```python
from build123d import *

# Parameters (mm, degrees)
SKETCH1_R               = 19.05
BOSS_EXTRUDE1_DEPTH     = 10.16
SKETCH2_R               = 6.35
CUT_EXTRUDE1_DEPTH      = 15.494
SKETCH6_W               = 12.7
SKETCH6_H               = 12.7
BOSS_EXTRUDE6_DEPTH     = 10.16
BOSS_EXTRUDE7_START     = -10.16
BOSS_EXTRUDE7_DEPTH     = 10.16
CIRPATTERN7_START       = -6.35
CIRPATTERN7_OUTLINE_W   = 10.16
CIRPATTERN7_OUTLINE_H   = 12.7
CIRPATTERN7_DEPTH       = 12.7
CIRPATTERN7_START_2     = -19.05
CIRPATTERN7_2_OUTLINE_W = 10.16
CIRPATTERN7_2_OUTLINE_H = 12.7
CIRPATTERN7_2_DEPTH     = 1.089487758
CIRPATTERN7_START_3     = 17.960512242
CIRPATTERN7_3_OUTLINE_W = 10.16
CIRPATTERN7_3_OUTLINE_H = 12.7
CIRPATTERN7_3_DEPTH     = 1.089487758
SKETCH7_W               = 12.7
SKETCH7_H               = 10.16
BOSS_EXTRUDE9_DEPTH     = 12.7
SKETCH10_W              = 12.7
SKETCH10_H              = 10.16
BOSS_EXTRUDE10_DEPTH    = 12.7
SKETCH11_W              = 12.7
SKETCH11_H              = 10.16
BOSS_EXTRUDE11_DEPTH    = 12.7
SKETCH12_R              = 3.302
CUT_EXTRUDE3_DEPTH      = 16.256
CIRPATTERN8_COUNT       = 4


# Read off the part's stored shape, not the designer's step: CirPattern7
with BuildPart() as part:
    # Sketch1 → Boss-Extrude1 (new body)
    with BuildSketch(Plane(origin=(0, 0, 0), x_dir=(1, 0, 0), z_dir=(0, 1, 0))):
        with Locations(Location((0, 0, 0), (0, 0, 270))):
            Circle(SKETCH1_R)
    extrude(amount=BOSS_EXTRUDE1_DEPTH)

    # Sketch2 → Cut-Extrude1 (cut)
    with BuildSketch(Plane(origin=(0, 10.16, 0), x_dir=(1, 0, 0), z_dir=(0, 1, 0))):
        with Locations(Location((0, 0, 0), (0, 0, 270))):
            Circle(SKETCH2_R)
    extrude(amount=-CUT_EXTRUDE1_DEPTH, mode=Mode.SUBTRACT)



with BuildPart() as body_2:
    # Sketch6 → Boss-Extrude6 (new body)
    with BuildSketch(Plane(origin=(0, 10.16, 0), x_dir=(1, 0, 0), z_dir=(0, 1, 0))):
        with Locations((0, -25.4)):
            Rectangle(SKETCH6_W, SKETCH6_H)
    extrude(amount=-BOSS_EXTRUDE6_DEPTH)


with BuildPart() as part_1:
    add(part.part)

    add(body_2.part)  # Boss-Extrude7 merges body 2
    # Sketch6<4> → Boss-Extrude7 (add)
    with BuildSketch(Plane(origin=(0, 10.16, 0), x_dir=(1, 0, 0), z_dir=(0, 1, 0)).offset(BOSS_EXTRUDE7_START)):
        with BuildLine():
            Line((-6.35, -17.960512242), (-6.35, -19.05))
            Line((-6.35, -19.05), (0, -19.05))
            ThreePointArc((0, -19.05), (-3.221392695, -18.775652561), (-6.35, -17.960512242))
        make_face()
        with BuildLine():
            ThreePointArc((6.35, -17.960512242), (3.221392695, -18.775652561), (0, -19.05))
            Line((0, -19.05), (6.35, -19.05))
            Line((6.35, -19.05), (6.35, -17.960512242))
        make_face()
    extrude(amount=BOSS_EXTRUDE7_DEPTH)

    # CirPattern7 outline → CirPattern7 (add)
    with BuildSketch(Plane.YZ.offset(CIRPATTERN7_START)):
        with Locations((5.08, -12.7)):
            Rectangle(CIRPATTERN7_OUTLINE_W, CIRPATTERN7_OUTLINE_H)
    extrude(amount=CIRPATTERN7_DEPTH)

    # CirPattern7 2 outline → CirPattern7 2 (add)
    with BuildSketch(Plane.YZ.offset(CIRPATTERN7_START_2)):
        with Locations((5.08, 0)):
            Rectangle(CIRPATTERN7_2_OUTLINE_W, CIRPATTERN7_2_OUTLINE_H)
    extrude(amount=CIRPATTERN7_2_DEPTH)

    # CirPattern7 3 outline → CirPattern7 3 (add)
    with BuildSketch(Plane.YZ.offset(CIRPATTERN7_START_3)):
        with Locations((5.08, 0)):
            Rectangle(CIRPATTERN7_3_OUTLINE_W, CIRPATTERN7_3_OUTLINE_H)
    extrude(amount=CIRPATTERN7_3_DEPTH)

    # Sketch7 → Boss-Extrude9 (add)
    with BuildSketch(Plane.ZY.offset(19.05)):
        with Locations((0, 5.08)):
            Rectangle(SKETCH7_W, SKETCH7_H)
    extrude(amount=BOSS_EXTRUDE9_DEPTH)

    # Sketch10 → Boss-Extrude10 (add)
    with BuildSketch(Plane(origin=(19.05, 0, 0), x_dir=(0, 0, -1), z_dir=(1, 0, 0))):
        with Locations((0, 5.08)):
            Rectangle(SKETCH10_W, SKETCH10_H)
    extrude(amount=BOSS_EXTRUDE10_DEPTH)

    # Sketch11 → Boss-Extrude11 (add)
    with BuildSketch(Plane(origin=(0, 0, -19.05), x_dir=(-1, 0, 0), z_dir=(0, 0, -1))):
        with Locations((0, 5.08)):
            Rectangle(SKETCH11_W, SKETCH11_H)
    extrude(amount=BOSS_EXTRUDE11_DEPTH)

    # Sketch12 → Cut-Extrude3 (cut)
    with BuildSketch(Plane.XY.offset(6.35)):
        with Locations((26.67, 5.08)):
            Circle(SKETCH12_R)
    cut_extrude3 = extrude(amount=-CUT_EXTRUDE3_DEPTH, mode=Mode.SUBTRACT)

    # CirPattern8: Cut-Extrude3 ×4 about axis
    cirpattern8_axis = Axis((0, 0, 0), (0, -1, 0))
    for i in range(1, CIRPATTERN8_COUNT):
        add(cut_extrude3.rotate(cirpattern8_axis, i * 360 / CIRPATTERN8_COUNT), mode=Mode.SUBTRACT)


solid = part_1.part
```
Check sheet for the modelled part. Datum: model origin and axes. Units: mm. A direction names the side the tool comes from. Round coordinates to 2 decimals unless told otherwise and drop trailing zeros. Loops run counter-clockwise (first coordinate to the right, second up) from the corner with the lowest first, then second, coordinate; pieces in that order, holes last. Notation, with made-up numbers: (-31.5, 19) - (-20.5, 19) arc R17 ccw to (-20.5, 42) - close; hole circle Ø10 at (-37, 56.5). An arc over 180 degrees is marked (long way). Answer as a JSON object with one key per item and string values. Group by question number.
Q1. Sectioned sample at C-C, the plane z = 0. Enter the section's corners in (x, y).
Q2. Mould release check, pull along X, two halves, no side actions. Record for faces 6 (the face through (6.35, 6, 23)), 7 (the face through (23.37, 5.23, 0.09)), 8 (the face through (-0.09, 5.23, 23.37)): released by +X, released by -X, zero draft, split by the parting line, or undercut.
Q3. Set-up check for faces 1 (the face through (-23, 5, 6.35)), 2 (the face through (23, 5, 6.35)), 3 (the face through (-5, 10.16, 5)), 4 (the face through (-6.35, 5, -23)), 5 (the face through (13.55, 5.01, -13.39)): record each of +Z, -Z, +X, -X, +Y, -Y from which the full face is reachable in a straight line by a thin tool's end or side.
Q4. Sectioned sample at A-A, the plane y = 5.08. Count the separate pieces of the cut face and the enclosed holes in it, plus the area to 3 significant figures.
Q5. Scan lines: line 1 along Z through (x, y) = (0, 2.5); line 2 along Y through (x, z) = (0.75, -26.67); line 3 along X through (y, z) = (3, 0). Record each from-to range of solid material in increasing order. Write a range as [from, to].
Q6. Sectioned sample at D-D, the plane z = 26.67. Enter the section's corners in (x, y), plus the area to 3 significant figures.
Q7. Sectioned sample at B-B, the plane x = 0. Enter the section's corners in (y, z), plus the area to 3 significant figures.
Q8. Gauge pin test, flat ends, axial feed: P1, Ø5, axis at x = 25.5, y = 3.5, coming from the +Z side; P2, Ø2, axis at x = 24, y = 9, coming from the -Z side; P3, Ø5, axis at y = 6.5, z = 25.5, coming from the +X side. Record the tip position at first contact, or that the pin passes through.
Solution:
{
 "1": {"outline": "(-31.75, 0) - (-6.35, 0) - (-6.35, 10.16) - (-31.75, 10.16) - close; (6.35, 0) - (31.75, 0) - (31.75, 10.16) - (6.35, 10.16) - close; hole circle Ø6.6 at (-26.67, 5.08); hole circle Ø6.6 at (26.67, 5.08)"},
 "2": {"face 6": "released by +X", "face 7": "undercut", "face 8": "zero draft"},
 "3": {"face 1": "+Z, -X, +Y, -Y", "face 2": "+Z, +X, +Y, -Y", "face 3": "+Z, -Z, +X, -X, +Y", "face 4": "-Z, -X, +Y, -Y", "face 5": "-Z, +X, +Y, -Y"},
 "4": {"separate pieces": "5", "enclosed holes": "1", "area": "1,340 mm²"},
 "5": {"line 1": "z = [-31.75, -28.73], [-24.61, -6.35], [6.35, 24.61], [28.73, 31.75]", "line 2": "y = [0, 1.78], [8.38, 10.16]", "line 3": "x = [-31.75, -29.23], [-24.11, -6.35], [6.35, 24.11], [29.23, 31.75]"},
 "6": {"outline": "(-6.35, 0) - (6.35, 0) - (6.35, 1.78) - (-6.35, 1.78) - close; (-6.35, 8.38) - (6.35, 8.38) - (6.35, 10.16) - (-6.35, 10.16) - close", "area": "45.2 mm²"},
 "7": {"outline": "(0, -31.75) - (10.16, -31.75) - (10.16, -6.35) - (0, -6.35) - close; (0, 6.35) - (10.16, 6.35) - (10.16, 31.75) - (0, 31.75) - close; hole circle Ø6.6 at (5.08, -26.67); hole circle Ø6.6 at (5.08, 26.67)", "area": "448 mm²"},
 "8": {"P1": "stops at z = 6.35", "P2": "stops at z = -6.35", "P3": "stops at x = 6.35"}
}
